Geometry check sheet. Reference: the model listing, model coordinates, mm. A direction names the side the tool comes from. Round coordinates to 2 decimals unless told otherwise and drop trailing zeros. Write each loop counter-clockwise with the first axis right and the second up, starting at its lowest first coordinate (ties: lowest second). Pieces come first, ordered by that corner, then holes. Notation, with made-up numbers: M 6,-33.5 L 52,-33.5 A20 cw 52,-28.5 Z; hole C 56.25,50 d6. An arc over 180 degrees is marked long. Put each result on its own line as item: value. Start each with the question number.
(1) Section check B-B on z = 17.5. Record the cut outline in (x, y) (3 decimals), then the cut area to 3 significant figures.
(2) Tool access check on faces 1 (the flat face through (0, 3.175, 1)), 2 (the flat face through (0, 0, -28)). Record the directions out of +Z, -Z, +X, -X, +Y, -Y that give a thin tool (end or side, any length) a straight path to the whole face; none if there is none.
(3) Gauge pin test, flat ends, axial feed: pin 1 (14.5 mm diameter, centred on x = -12.47, z = 46.23, fed in from +Y) (3 decimals); pin 2 (1.8 mm diameter, centred on x = -1.5, z = -23.75, fed in from -Y). Record the tip position at first contact, or that the pin passes through.
(4) Material ranges on probe 1 along X at (y, z) = (0.75, -31.5); probe 2 along Z at (x, y) = (-21, 1.5); probe 3 along Z at (x, y) = (-16.5, -0.5), recorded low to high.
(5) Section check D-D on y = -1.75. Record the cut outline in (x, z), then the cut area to 3 significant figures.
(6) Section check C-C on x = -16.5. Record the cut outline in (y, z) (3 decimals), then the cut area to 3 significant figures.
(7) Section check A-A on x = -1.5. Record the cut outline in (y, z) (3 decimals), then the cut area to 3 significant figures.
(8) Mould release check, pull along X, two halves, no side actions. Record for faces 3 (the flat face through (35.645, 0, -1)), 4 (the cylindrical face through (-24.08, 0.04, 19.53)), 5 (the flat face through (0, 0, 55.294)): pulls with the +X half, pulls with the -X half, needs draft (parallel to the pull), parting line crosses it, or undercut.
from build123d import *

# Parameters (mm, degrees)
F0_W     = 71.2898522615
F0_H     = 110.58742553
F0_R     = 5.8240303567
F0_R_2   = 5.544554678
F0_R_3   = 5.5476903885
F0_R_4   = 4.7529819841
F1_DEPTH = 3.175
F2_DEPTH = 3.175


with BuildPart() as f1:
    # F0 (on Front) → F1 (new body, symmetric)
    with BuildSketch(Plane.XZ):
        Rectangle(F0_W, F0_H)
        with BuildLine():
            ThreePointArc((-2.9955138452, -23.9786170423), (-1.4977569226, -22.2334064032), (0, -23.9786170423))
            Line((0, -23.9786170423), (0, -32.0213139057))
            ThreePointArc((0, -32.0213139057), (-1.4977569226, -33.8227026245), (-2.9955138452, -32.0213139057))
            Line((-2.9955138452, -32.0213139057), (-2.9955138452, -23.9786170423))
        make_face(mode=Mode.SUBTRACT)
        with Locations((-18.2633008808, 19.2709285766)):
            Circle(F0_R, mode=Mode.SUBTRACT)
        with Locations((-25.2595208585, 35.7538498938)):
            Circle(F0_R_2, mode=Mode.SUBTRACT)
        with Locations((-12.4694257975, 46.225041151)):
            Circle(F0_R_3, mode=Mode.SUBTRACT)
        with Locations((14.4846877083, 21.0342817008)):
            Circle(F0_R_4, mode=Mode.SUBTRACT)
    extrude(amount=F1_DEPTH, both=True)

    # F0 (on Front) → F2 (join, symmetric)
    with BuildSketch(Plane.XZ):
        Rectangle(F0_W, F0_H)
        with BuildLine():
            ThreePointArc((-2.9955138452, -23.9786170423), (-1.4977569226, -22.2334064032), (0, -23.9786170423))
            Line((0, -23.9786170423), (0, -32.0213139057))
            ThreePointArc((0, -32.0213139057), (-1.4977569226, -33.8227026245), (-2.9955138452, -32.0213139057))
            Line((-2.9955138452, -32.0213139057), (-2.9955138452, -23.9786170423))
        make_face(mode=Mode.SUBTRACT)
        with Locations((-18.2633008808, 19.2709285766)):
            Circle(F0_R, mode=Mode.SUBTRACT)
        with Locations((-25.2595208585, 35.7538498938)):
            Circle(F0_R_2, mode=Mode.SUBTRACT)
        with Locations((-12.4694257975, 46.225041151)):
            Circle(F0_R_3, mode=Mode.SUBTRACT)
        with Locations((14.4846877083, 21.0342817008)):
            Circle(F0_R_4, mode=Mode.SUBTRACT)
    extrude(amount=F2_DEPTH, both=True)


solid = f1.part
Answers follow:
1. outline: M -35.645,-3.175 L -23.812,-3.175 L -23.812,3.175 L -35.645,3.175 Z; M -12.715,-3.175 L 11.307,-3.175 L 11.307,3.175 L -12.715,3.175 Z; M 17.663,-3.175 L 35.645,-3.175 L 35.645,3.175 L 17.663,3.175 Z
1. area: 342 mm^2
2. face 1: +Z, -Z, +X, -X, +Y
2. face 2: +Y, -Y
3. pin 1: stops at y = 3.175
3. pin 2: passes through
4. probe 1: x = -35.64 to -3, 0 to 35.64
4. probe 2: z = -55.29 to 14.13, 24.41 to 32.2, 39.3 to 55.29
4. probe 3: z = -55.29 to 13.72, 24.82 to 42.41, 50.04 to 55.29
5. outline: M -35.64,-55.29 L 35.64,-55.29 L 35.64,55.29 L -35.64,55.29 Z; hole C -25.26,35.75 d11.09; hole C -18.26,19.27 d11.65; hole C -12.47,46.23 d11.1; hole M -3,-32.02 A1.52 ccw long 0,-32.02 L 0,-23.98 A1.52 ccw long -3,-23.98 Z; hole C 14.48,21.03 d9.51
5. area: 7,480 mm^2
6. outline: M -3.175,-55.294 L 3.175,-55.294 L 3.175,13.72 L -3.175,13.72 Z; M -3.175,24.822 L 3.175,24.822 L 3.175,42.413 L -3.175,42.413 Z; M -3.175,50.037 L 3.175,50.037 L 3.175,55.294 L -3.175,55.294 Z
6. area: 583 mm^2
7. outline: M -3.175,-55.294 L 3.175,-55.294 L 3.175,-33.823 L -3.175,-33.823 Z; M -3.175,-22.233 L 3.175,-22.233 L 3.175,55.294 L -3.175,55.294 Z
7. area: 629 mm^2
8. face 3: pulls with the +X half
8. face 4: undercut
8. face 5: needs draft
